from build123d import *

# Parameters (mm, degrees)
BOSS_EXTRUDE1_DEPTH  = 132.4
SKETCH3_R            = 4.75
BOSS_EXTRUDE2_DEPTH  = 1
CUT_EXTRUDE1_DEPTH   = 1
CUT_EXTRUDE1_DRAFT   = 1
MIRROR1_COPY_1_DEPTH = 1
MIRROR1_COPY_1_DRAFT = 1


with BuildPart() as part:
    # Sketch2 → Boss-Extrude1 (new body)
    with BuildSketch(Plane.XY):
        with BuildLine():
            Line((-1.225, 1.828623949), (1.225, 1.828623949))
            Line((1.225, 1.828623949), (1.225, 3.278623949))
            ThreePointArc((1.225, 3.278623949), (0, -3.5), (-1.225, 3.278623949))
            Line((-1.225, 3.278623949), (-1.225, 1.828623949))
        make_face()
    extrude(amount=BOSS_EXTRUDE1_DEPTH)

    # Sketch3 → Boss-Extrude2 (add)
    with BuildSketch(Plane(origin=(0, 0, 0), x_dir=(-1, 0, 0), z_dir=(0, 0, -1))):
        Circle(SKETCH3_R)
    boss_extrude2 = extrude(amount=BOSS_EXTRUDE2_DEPTH)

    # Sketch4 → Revolve1 (revolve)
    with BuildSketch(Plane(origin=(0, 0, 0), x_dir=(1, 0, 0), z_dir=(0, 1, 0))):
        with BuildLine():
            Line((0, 1), (4.75, 1))
            ThreePointArc((4.75, 1), (3.358757211, 4.358757211), (0, 5.75))
            Line((0, 5.75), (0, 1))
        make_face()
    revolve1 = revolve(axis=Axis((0, 0, -5.75), (0, 0, 1)))


with BuildPart() as cut_extrude1_tool:
    # Sketch5 → Cut-Extrude1 (with draft: the straight prism first)
    with BuildSketch(Plane(origin=(0, 0, -5.75), x_dir=(-1, 0, 0), z_dir=(0, 0, -1))):
        Polygon((0, 1.6), (-0.3, 1.3), (-0.3, 0.3), (-1.3, 0.3), (-1.6, 0), (-1.3, -0.3), (-0.3, -0.3), (-0.3, -1.3), (0, -1.6), (0.3, -1.3), (0.3, -0.3), (1.3, -0.3), (1.6, 0), (1.3, 0.3), (0.3, 0.3), (0.3, 1.3), align=None)
    extrude(amount=-CUT_EXTRUDE1_DEPTH)
    # Cut-Extrude1: the draft: its side faces are tilted about the plane it starts from
    cut_extrude1_sides = [cut_extrude1_tool.faces().sort_by_distance(p)[0] for p in [
        (0.15, 1.45, -5.25),
        (0.3, 0.8, -5.25),
        (0.8, 0.3, -5.25),
        (1.45, 0.15, -5.25),
        (1.45, -0.15, -5.25),
        (0.8, -0.3, -5.25),
        (0.3, -0.8, -5.25),
        (0.15, -1.45, -5.25),
        (-0.15, -1.45, -5.25),
        (-0.3, -0.8, -5.25),
        (-0.8, -0.3, -5.25),
        (-1.45, -0.15, -5.25),
        (-1.45, 0.15, -5.25),
        (-0.8, 0.3, -5.25),
        (-0.3, 0.8, -5.25),
        (-0.15, 1.45, -5.25),
    ]]
    draft(cut_extrude1_sides, Plane(origin=(0, 0, -5.75), x_dir=(-1, 0, 0), z_dir=(0, 0, -1)), CUT_EXTRUDE1_DRAFT)


with BuildPart() as part_1:
    add(part.part)

    # Cut-Extrude1: cut by cut_extrude1_tool
    add(cut_extrude1_tool.part, mode=Mode.SUBTRACT)

    # Mirror1: Boss-Extrude2, Revolve1 across plane
    add(boss_extrude2.mirror(Plane.XY.offset(66.2)))
    add(revolve1.mirror(Plane.XY.offset(66.2)))


with BuildPart() as mirror1_copy_1_tool:
    # Mirror1 copy 1 sketch → Mirror1 copy 1 (with draft: the straight prism first)
    with BuildSketch(Plane(origin=(0, 0, 138.15), x_dir=(-1, 0, 0), z_dir=(0, 0, 1))):
        Polygon((0, -1.6), (-0.3, -1.3), (-0.3, -0.3), (-1.3, -0.3), (-1.6, 0), (-1.3, 0.3), (-0.3, 0.3), (-0.3, 1.3), (0, 1.6), (0.3, 1.3), (0.3, 0.3), (1.3, 0.3), (1.6, 0), (1.3, -0.3), (0.3, -0.3), (0.3, -1.3), align=None)
    extrude(amount=-MIRROR1_COPY_1_DEPTH)
    # Mirror1 copy 1: the draft: its side faces are tilted about the plane it starts from
    mirror1_copy_1_sides = [mirror1_copy_1_tool.faces().sort_by_distance(p)[0] for p in [
        (0.15, 1.45, 137.65),
        (0.3, 0.8, 137.65),
        (0.8, 0.3, 137.65),
        (1.45, 0.15, 137.65),
        (1.45, -0.15, 137.65),
        (0.8, -0.3, 137.65),
        (0.3, -0.8, 137.65),
        (0.15, -1.45, 137.65),
        (-0.15, -1.45, 137.65),
        (-0.3, -0.8, 137.65),
        (-0.8, -0.3, 137.65),
        (-1.45, -0.15, 137.65),
        (-1.45, 0.15, 137.65),
        (-0.8, 0.3, 137.65),
        (-0.3, 0.8, 137.65),
        (-0.15, 1.45, 137.65),
    ]]
    draft(mirror1_copy_1_sides, Plane(origin=(0, 0, 138.15), x_dir=(-1, 0, 0), z_dir=(0, 0, 1)), MIRROR1_COPY_1_DRAFT)


with BuildPart() as part_2:
    add(part_1.part)

    # Mirror1 copy 1: cut by mirror1_copy_1_tool
    add(mirror1_copy_1_tool.part, mode=Mode.SUBTRACT)


solid = part_2.part
The model under review builds one solid part; all positions refer to its coordinate system, in mm. A direction names the side the tool comes from. Round coordinates to 2 decimals unless told otherwise and drop trailing zeros. Order: outer loops, then holes, each group sorted by start corner. A loop starts at its lowest first (then second) coordinate and runs counter-clockwise, first axis right, second up. Notation, with made-up numbers: (-7, -6.5) -> (30, -6.5) arc R7 ccw to (30, -1.5) -> close; hole circle Ø3 at (-11, 14). An arc over 180 degrees is marked (long way). Return JSON: item names as keys, results as strings.
1. The part is to be moulded in two halves that separate along Z. For faces 1 (the face through (-2.192, -4.214, 132.893)), 2 (the face through (0.1, -3.5, 65.3)), 3 (the face through (0, 2, 0)), say which applies: +Z half, -Z half, draft (parallel to the pull), parting line (faces both ways), or undercut.
Answer block:
{"face 1": "draft", "face 2": "undercut", "face 3": "undercut"}
2. Take a section at A-A (z = 106.5). Write out the cut boundary in (x, y) (3 decimals).
Answer block:
{"outline": "(-1.225, 1.829) -> (-1.225, 3.279) arc R3.5 ccw (long way) to (1.225, 3.279) -> (1.225, 1.829) -> close"}
3. For faces 4 (the face through (-2.192, -4.214, -0.493)), 5 (the face through (0, 2, 132.4)), 6 (the face through (0, 1.829, 65)), list the 3-axis set-ups (+Z, -Z, +X, -X, +Y, -Y) from which the entire face can be reached by the end or side of a thin tool; tool diameter is ignored.
Answer block:
{"face 4": "+Z, -Z", "face 5": "none", "face 6": "+Y"}
4. Insertion check: P1, Ø4, axis at x = -0.5, y = 3.5, coming from the -Z side; P2, Ø3, axis at x = -1, z = 22.5, coming from the -Y side; P3, Ø0.7, axis at y = 2.5, z = 58, coming from the +X side. Each pin has a flat end and moves straight along its axis. Give the tip position at first contact, or say it passes through.
Answer block:
{"P1": "stops at z = -5.49", "P2": "stops at y = -3.5", "P3": "stops at x = 2.76"}
5. For L1, parallel to X at y = 0, z = 87.5; L2, parallel to Z at x = -1, y = 0; L3, parallel to X at y = 2.75, z = 60 (3 decimals), list the stretches that pass through material, from the lowest coordinate up. Write a range as [from, to].
Answer block:
{"L1": "x = [-3.5, 3.5]", "L2": "z = [-4.75, 137.15]", "L3": "x = [-2.165, -1.225], [1.225, 2.165]"}
